```python
from build123d import *

# Parameters (mm, degrees)
F2_DEPTH = 25.4
F3_R     = 6.349176
F4_DEPTH = 25.401
F6_DEPTH = 23.465528
F7_W     = 44.45
F7_H     = 25.4
F8_DEPTH = 12.7


with BuildPart() as f2:
    # F1 (on face) → F2 (new body)
    with BuildSketch(Plane.XZ):
        with BuildLine():
            Line((11.798794, 39.917438), (-32.651206, 39.917438))
            ThreePointArc((-32.651206, 39.917438), (-35.515616, 50.065544), (-45.058145, 54.552085))
            Line((-45.058145, 54.552085), (-45.347569, 54.552085))
            ThreePointArc((-45.347569, 54.552085), (-53.956125, 51.054556), (-57.87898, 42.631305))
            Line((-57.87898, 42.631305), (-57.87898, 16.452909))
            Line((-57.87898, 16.452909), (11.716359, 16.452909))
            Line((11.716359, 16.452909), (11.798794, 30.775242))
            Line((11.798794, 30.775242), (11.798794, 39.917438))
        make_face()
    extrude(amount=F2_DEPTH)

    # F3 (on face) → F4 (cut, through all)
    with BuildSketch(Plane.XZ.offset(25.4)):
        with Locations((-45.202857, 41.852909)):
            Circle(F3_R)
    extrude(amount=-F4_DEPTH, mode=Mode.SUBTRACT)

    # F5 (on face) → F6 (cut, through all)
    with BuildSketch(Plane.XY.offset(39.917438)):
        with BuildLine():
            Line((-19.951206, -12.7), (-19.951206, -6.35))
            ThreePointArc((-19.951206, -6.35), (-26.301206, -12.7), (-19.951206, -19.05))
            Line((-19.951206, -19.05), (-19.951206, -12.7))
        make_face()
        with BuildLine():
            ThreePointArc((-13.601206, -12.7), (-15.461078, -8.209872), (-19.951206, -6.35))
            Line((-19.951206, -6.35), (-19.951206, -12.7))
            Line((-19.951206, -12.7), (-19.951206, -19.05))
            ThreePointArc((-19.951206, -19.05), (-15.461078, -17.190128), (-13.601206, -12.7))
        make_face()
        with BuildLine():
            ThreePointArc((-0.901206, -19.05), (-7.251206, -12.7), (-0.901206, -6.35))
            Line((-0.901206, -6.35), (-19.951206, -6.35))
            ThreePointArc((-19.951206, -6.35), (-15.461078, -8.209872), (-13.601206, -12.7))
            ThreePointArc((-13.601206, -12.7), (-15.461078, -17.190128), (-19.951206, -19.05))
            Line((-19.951206, -19.05), (-0.901206, -19.05))
        make_face()
        with BuildLine():
            ThreePointArc((-0.901206, -19.05), (3.588922, -17.190128), (5.448794, -12.7))
            ThreePointArc((5.448794, -12.7), (3.588922, -8.209872), (-0.901206, -6.35))
            ThreePointArc((-0.901206, -6.35), (-7.251206, -12.7), (-0.901206, -19.05))
        make_face()
    extrude(amount=-F6_DEPTH, mode=Mode.SUBTRACT)

    # F7 (on face) → F8 (cut)
    with BuildSketch(Plane.XY.offset(39.917438)):
        with Locations((-10.426206, -12.7)):
            Rectangle(F7_W, F7_H)
    extrude(amount=-F8_DEPTH, mode=Mode.SUBTRACT)


solid = f2.part
```
Can you work these out from the model? Positions are in its coordinate system, mm. A direction names the side the tool comes from. Coordinates: 2 decimals unless noted, no trailing zeros. Loops run counter-clockwise (first coordinate to the right, second up) from the corner with the lowest first, then second, coordinate; pieces in that order, holes last. Notation, with made-up numbers: (53.25, 0) - (67.25, 0) arc R17 cw to (67.25, 27) - close; hole circle Ø5 at (76.5, 61). An arc over 180 degrees is marked (long way). Use a Markdown table: item, result.
Item 1: For faces 1 (the face through (-32.651, -13, 34)), 2 (the face through (-11, -19.05, 22)), 3 (the face through (-39, -25.4, 32)), which set-ups out of +Z, -Z, +X, -X, +Y, -Y let a thin tool reach every point of the face, with its end or its side?
Numbers:
| item | result |
|---|---|
| face 1 | +X, +Y, -Y |
| face 2 | +Z, -Z |
| face 3 | +Z, -Z, +X, -X, -Y |
Item 2: We'd pull the mould along Z, two halves only. Please class faces 4 (the face through (-26.3, -12.6, 21.9)), 5 (the face through (-53.859, -12.522, 51.146)), 6 (the face through (-51.546, -12.878, 42.132)): released by +Z, released by -Z, zero draft, split by the parting line, or undercut.
Numbers:
| item | result |
|---|---|
| face 4 | zero draft |
| face 5 | released by +Z |
| face 6 | undercut |
Item 3: I want a section at C-C on z = 36.5. Please give me the cut outline in (x, y), and give its area (3 significant figures).
Numbers:
| item | result |
|---|---|
| outline | (-57.88, -25.4) - (-48.62, -25.4) - (-48.62, 0) - (-57.88, 0) - close; (-41.79, -25.4) - (-32.65, -25.4) - (-32.65, 0) - (-41.79, 0) - close |
| area | 467 mm2 |
Item 4: I want a section at D-D on y = -11.25. Please give me the cut outline in (x, z), and give its area (3 significant figures).
Numbers:
| item | result |
|---|---|
| outline | (-57.88, 16.45) - (-26.13, 16.45) - (-26.13, 27.22) - (-32.65, 27.22) - (-32.65, 39.92) arc R12.7 ccw to (-45.06, 54.55) - (-45.35, 54.55) arc R12.7 ccw to (-57.88, 42.63) - close; (5.28, 16.45) - (11.72, 16.45) - (11.78, 27.22) - (5.28, 27.22) - close; hole circle Ø12.7 at (-45.2, 41.85) |
| area | 907 mm2 |
Item 5: If I drill on probe 1 along X at (y, z) = (-20.25, 25.5); probe 2 along X at (y, z) = (-8.5, 37); probe 3 along Z at (x, y) = (-15.5, -24), over which ranges is the centre line in solid material (lowest first)? Write a range as from..to.
Numbers:
| item | result |
|---|---|
| probe 1 | x = -57.88..11.77 |
| probe 2 | x = -57.88..-49.3, -41.11..-32.65 |
| probe 3 | z = 16.45..27.22 |
Item 6: I want a section at B-B on x = -11.5. Please give me the cut outline in (y, z).
Numbers:
| item | result |
|---|---|
| outline | (-25.4, 16.45) - (-19.05, 16.45) - (-19.05, 27.22) - (-25.4, 27.22) - close; (-6.35, 16.45) - (0, 16.45) - (0, 27.22) - (-6.35, 27.22) - close |
Item 7: I want a section at A-A on y = -14.5. Please give me the cut outline in (x, z), and give its area (3 significant figures).
Numbers:
| item | result |
|---|---|
| outline | (-57.88, 16.45) - (-26.04, 16.45) - (-26.04, 27.22) - (-32.65, 27.22) - (-32.65, 39.92) arc R12.7 ccw to (-45.06, 54.55) - (-45.35, 54.55) arc R12.7 ccw to (-57.88, 42.63) - close; (5.19, 16.45) - (11.72, 16.45) - (11.78, 27.22) - (5.19, 27.22) - close; hole circle Ø12.7 at (-45.2, 41.85) |
| area | 909 mm2 |
Item 8: Will these pins go through, and if not, where does the flat tip stop? pin 1 (1 mm diameter, centred on x = -9.5, y = -4.5, fed in from +Z); pin 2 (10 mm diameter, centred on y = -7.5, z = 36.5, fed in from +X); pin 3 (8 mm diameter, centred on x = -50, y = -14.5, fed in from +Z).
Numbers:
| item | result |
|---|---|
| pin 1 | stops at z = 27.22 |
| pin 2 | stops at x = -32.51 |
| pin 3 | stops at z = 54.53 |
